Model file for the job. Use its own axes, mm. Face numbers are marked on the shaded views. A direction names the side the tool comes from. Round coordinates to 2 decimals unless told otherwise and drop trailing zeros. Order: outer loops, then holes, each group sorted by start corner. A loop starts at its lowest first (then second) coordinate and runs counter-clockwise, first axis right, second up. Notation, with made-up numbers: (75, 4.25) -> (85, 4.25) arc R23 ccw to (85, 20.25) -> close; hole circle Ø11 at (84, -28.5). An arc over 180 degrees is marked (long way). Put each result on its own line as item: value. Start each with the question number.
Q1. Cut at C-C, the plane z = -7.25. List the corners of the cut face in (x, y).
Q2. Cut at B-B, the plane x = 3.75. List the corners of the cut face in (y, z).
Q3. Probe L1, parallel to Y at x = 0, z = 3.5; L2, parallel to Z at x = -5, y = -25; L3, parallel to Y at x = 3.75, z = -15.5. List the from-to ranges inside material, lowest first.
Q4. Flat gauge pins, fed straight in: P1, Ø4, axis at y = -59, z = -14.5, coming from the -X side; P2, Ø9, axis at x = 2, z = -14.5, coming from the +Y side; P3, Ø3.5, axis at x = 0, y = 57.5, coming from the +Z side; P4, Ø4, axis at y = -61, z = -3.5, coming from the +X side. Where does each tip first touch, or does it go through?
Q5. Cut at A-A, the plane y = -49. List the corners of the cut face in (x, z).
Q6. Cut at D-D, the plane y = -35. List the corners of the cut face in (x, z).
Q7. 3-axis set-ups, long thin cutter, end or side, ignore diameter. For the marked faces 1, 2, 3 and 4: which of +Z, -Z, +X, -X, +Y, -Y reach the whole face in a straight line?
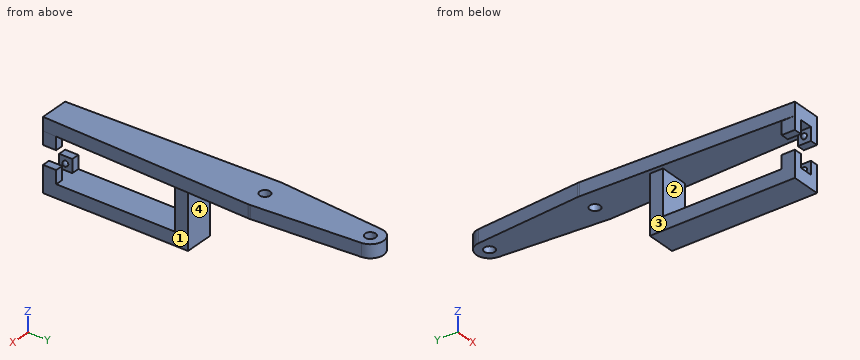
from build123d import *

# Parameters (mm, degrees)
SKETCH1_R           = 2
SKETCH1_R_2         = 5
BOSS_EXTRUDE1_DEPTH = 5
SKETCH2_W           = 11
SKETCH2_H           = 5
BOSS_EXTRUDE2_DEPTH = 5
SKETCH2_3_W         = 5.5
SKETCH2_3_H         = 5
BOSS_EXTRUDE3_DEPTH = 22
SKETCH4_W           = 5
SKETCH4_H           = 5
CUT_EXTRUDE1_DEPTH  = 20
SKETCH6_W           = 11
SKETCH6_H           = 5
BOSS_EXTRUDE4_DEPTH = 50


with BuildPart() as part:
    # Sketch1 → Boss-Extrude1 (new body)
    with BuildSketch(Plane.XY):
        with BuildLine():
            ThreePointArc((7.996084375, 17.249730801), (0, 9.5), (-7.996084375, 17.249730801))
            Line((-7.996084375, 17.249730801), (-5.5, -62.5))
            Line((-5.5, -62.5), (5.5, -62.5))
            Line((5.5, -62.5), (7.996084375, 17.249730801))
        make_face()
        with BuildLine():
            ThreePointArc((7.97746827, 18.1), (0, 25.5), (-7.97746827, 18.1))
            ThreePointArc((-7.97746827, 18.1), (-7.998083236, 17.675112958), (-7.996084375, 17.249730801))
            ThreePointArc((-7.996084375, 17.249730801), (0, 9.5), (7.996084375, 17.249730801))
            ThreePointArc((7.996084375, 17.249730801), (7.999021034, 17.374850086), (8, 17.5))
            ThreePointArc((8, 17.5), (7.994365083, 17.800211458), (7.97746827, 18.1))
        make_face()
        with Locations((0, 17.5)):
            Circle(SKETCH1_R, mode=Mode.SUBTRACT)
        with BuildLine():
            ThreePointArc((5, 57.5), (-0.187632161, 52.503521823), (-4.985917669, 57.875))
            Line((-4.985917669, 57.875), (-7.97746827, 18.1))
            ThreePointArc((-7.97746827, 18.1), (0, 25.5), (7.97746827, 18.1))
            Line((7.97746827, 18.1), (4.985917669, 57.875))
            ThreePointArc((4.985917669, 57.875), (4.996478177, 57.687632161), (5, 57.5))
        make_face()
        with Locations((0, 57.5)):
            Circle(SKETCH1_R_2)
        with Locations((0, 57.5)):
            Circle(SKETCH1_R, mode=Mode.SUBTRACT)
    extrude(amount=BOSS_EXTRUDE1_DEPTH)

    # Sketch2 → Boss-Extrude2 (add)
    with BuildSketch(Plane(origin=(0, 0, 0), x_dir=(-1, 0, 0), z_dir=(0, 0, -1))):
        with Locations((0, -60)):
            Rectangle(SKETCH2_W, SKETCH2_H)
    boss_extrude2 = extrude(amount=BOSS_EXTRUDE2_DEPTH)

    # Sketch2<3> → Boss-Extrude3 (add)
    with BuildSketch(Plane(origin=(0, 0, 0), x_dir=(-1, 0, 0), z_dir=(0, 0, -1))):
        with Locations((-2.75, -10)):
            Rectangle(SKETCH2_3_W, SKETCH2_3_H)
        with Locations((2.75, -10)):
            Rectangle(SKETCH2_3_W, SKETCH2_3_H)
    extrude(amount=BOSS_EXTRUDE3_DEPTH)

    # Sketch4 → Cut-Extrude1 (cut)
    with BuildSketch(Plane(origin=(0, -57.5, 0), x_dir=(1, 0, 0), z_dir=(0, 1, 0))):
        with Locations((0, 2.5)):
            Rectangle(SKETCH4_W, SKETCH4_H)
    cut_extrude1 = extrude(amount=-CUT_EXTRUDE1_DEPTH, mode=Mode.SUBTRACT)

    # Sketch5 → Revolve1 (revolve)
    with BuildSketch(Plane.ZY.offset(-2.5)):
        with BuildLine():
            Line((-3.5, -60), (-1.5, -60))
            ThreePointArc((-1.5, -60), (-2.5, -61), (-3.5, -60))
        make_face()
    revolve1 = revolve(axis=Axis((2.5, -60, 0), (0, 0, -1)))

    # Mirror1: Revolve1 across plane
    add(revolve1.mirror(Plane(origin=(0, 0, 0), x_dir=(0, 0, 1), z_dir=(1, 0, 0))))

    # Sketch6 → Boss-Extrude4 (add)
    with BuildSketch(Plane(origin=(0, -12.5, 0), x_dir=(-1, 0, 0), z_dir=(0, -1, 0))):
        with Locations((0, 19.5)):
            Rectangle(SKETCH6_W, SKETCH6_H)
    extrude(amount=BOSS_EXTRUDE4_DEPTH)

    # Mirror2: Boss-Extrude2, Cut-Extrude1, Revolve1 across plane
    add(boss_extrude2.mirror(Plane(origin=(0, 0, -8.5), x_dir=(1, 0, 0), z_dir=(0, 0, -1))))
    add(cut_extrude1.mirror(Plane(origin=(0, 0, -8.5), x_dir=(1, 0, 0), z_dir=(0, 0, -1))), mode=Mode.SUBTRACT)
    add(revolve1.mirror(Plane(origin=(0, 0, -8.5), x_dir=(1, 0, 0), z_dir=(0, 0, -1))))

    # Mirror2 copy 1 sketch → Mirror2 copy 1 (revolve)
    with BuildSketch(Plane(origin=(-2.5, 0, -17), x_dir=(0, 0, -1), z_dir=(1, 0, 0))):
        with BuildLine():
            Line((-3.5, -60), (-1.5, -60))
            ThreePointArc((-1.5, -60), (-2.5, -61), (-3.5, -60))
        make_face()
    revolve(axis=Axis((-2.5, -60, -17), (0, 0, 1)))


solid = part.part
Ans:
1. outline: (-5.5, -12.5) -> (5.5, -12.5) -> (5.5, -7.5) -> (-5.5, -7.5) -> close
2. outline: (-62.5, -22) -> (-7.5, -22) -> (-7.5, 0) -> (60.81, 0) -> (60.81, 5) -> (-62.5, 5) -> (-62.5, -5) -> (-57.5, -5) -> (-57.5, 0) -> (-12.5, 0) -> (-12.5, -17) -> (-57.5, -17) -> (-57.5, -12) -> (-62.5, -12) -> close
3. L1: y = -62.5 to 15.5, 19.5 to 55.5, 59.5 to 62.5
3. L2: z = -22 to -17, 0 to 5
3. L3: y = -62.5 to -57.5, -12.5 to -7.5
4. P1: stops at x = -5.5
4. P2: stops at y = -7.5
4. P3: passes through
4. P4: stops at x = 5.5
5. outline: (-5.92, 0) -> (5.92, 0) -> (5.92, 5) -> (-5.92, 5) -> close; (-5.5, -22) -> (5.5, -22) -> (5.5, -17) -> (-5.5, -17) -> close
6. outline: (-6.36, 0) -> (6.36, 0) -> (6.36, 5) -> (-6.36, 5) -> close; (-5.5, -22) -> (5.5, -22) -> (5.5, -17) -> (-5.5, -17) -> close
7. face 1: -Z, +X, +Y, -Y
7. face 2: +X, -X
7. face 3: -Z, -X, +Y, -Y
7. face 4: -Z, +X, -X, +Y
